Read the model definition and answer for the solid it produces. Units are mm, in the model's axes. Face numbers are marked on the shaded views. A direction names the side the tool comes from. Coordinates: 2 decimals unless noted, no trailing zeros. Loops run counter-clockwise (first coordinate to the right, second up) from the corner with the lowest first, then second, coordinate; pieces in that order, holes last.
from build123d import *

# Parameters (mm, degrees)
FILLET1_R       = 0.2
FILLET2_R       = 0.4
HEX_2_DEPTH     = 2
THDSCHPAT_COUNT = 29
THDSCHPAT_PITCH = 0.689655172


with BuildPart() as part:
    # BodySke → Base-Revolve (revolve)
    with BuildSketch(Plane.XY, mode=Mode.PRIVATE) as base_revolve_sk:
        Polygon((0, 0), (0, 3.5), (4, 3.5), (4, 2), (43.61, 2), (44, 1.61), (44, 0), align=None)
    revolve(base_revolve_sk.sketch.rotate(Axis((-31.75, 0, 0), (1, 0, 0)), 90), axis=Axis((-31.75, 0, 0), (1, 0, 0)))  # turned: the seam where the file's is

    # Fillet1
    fillet1_edges = [part.edges().sort_by_distance(p)[0] for p in [
        (4, 0, -2),
    ]]
    fillet(fillet1_edges, radius=FILLET1_R)

    # Fillet2
    fillet2_edges = [part.edges().sort_by_distance(p)[0] for p in [
        (0, 0, -3.5),
    ]]
    fillet(fillet2_edges, radius=FILLET2_R)

    # Sketch2 → Hex-PreBroach (revolve, cut)
    with BuildSketch(Plane.XY, mode=Mode.PRIVATE) as hex_prebroach_sk:
        Polygon((0, 1.51), (2, 1.51), (2.871798906, 0), (0, 0), align=None)
    revolve(hex_prebroach_sk.sketch.rotate(Axis((0, 0, 0), (1, 0, 0)), 90), axis=Axis((0, 0, 0), (1, 0, 0)), mode=Mode.SUBTRACT)  # turned: the seam where the file's is

    # Sketch3 → Hex 2 (cut)
    with BuildSketch(Plane(origin=(0, 0, 0), x_dir=(0, 0.5, 0.866025404), z_dir=(-1, 0, 0))):
        Polygon((0.871798906, 1.51), (-0.871798906, 1.51), (-1.743597813, 0), (-0.871798906, -1.51), (0.871798906, -1.51), (1.743597813, 0), align=None)
    extrude(amount=-HEX_2_DEPTH, mode=Mode.SUBTRACT)

    # ThdSchSke → ThreadSchematic (revolve, cut)
    with BuildSketch(Plane.XY, mode=Mode.PRIVATE) as threadschematic_sk:
        Polygon((24, -1.61), (23.72691906, -2), (23.72691906, -2.5), (24.27308094, -2.5), (24.27308094, -2), align=None)
    threadschematic = revolve(threadschematic_sk.sketch.rotate(Axis((-3.175, 0, 0), (1, 0, 0)), 270), axis=Axis((-3.175, 0, 0), (1, 0, 0)), mode=Mode.SUBTRACT)  # turned: the seam where the file's is

    # ThdSchPat: ThreadSchematic ×29
    with Locations(*[(i * THDSCHPAT_PITCH, 0, 0) for i in range(1, THDSCHPAT_COUNT)]):
        add(threadschematic, mode=Mode.SUBTRACT)


solid = part.part
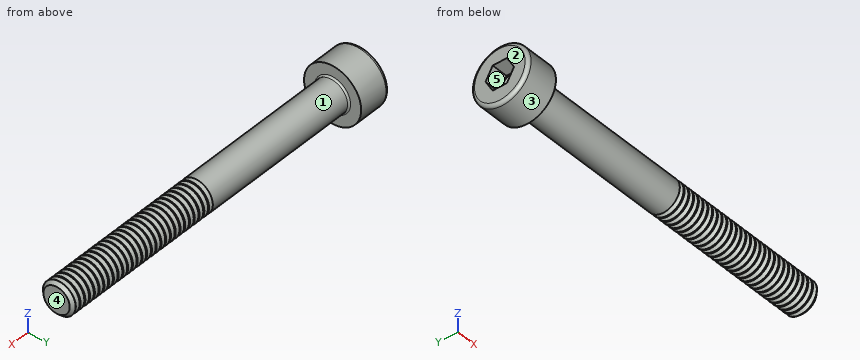
Q1. Flat-ended cylindrical pins translate along their axes: pin 1 Ø1 at (x, z) = (10, -0.5) entering from +Y; pin 2 Ø1.5 at (x, y) = (33, 1) entering from +Z; pin 3 Ø0.6 at (y, z) = (-0.5, -1) entering from -X. Find the tip coordinate at first contact, or state that the pin passes through.
Findings below:
pin 1: stops at y = 2
pin 2: stops at z = 1.98
pin 3: stops at x = 2.05
Q2. A cutting plane is placed at A-A (x = 9.5). Give the vertices of the cut face in (y, z).
Findings below:
outline: circle Ø4 at (0, 0)
Q3. Straight lines are drawn through the part: probe 1 along X at (y, z) = (-1.75, 1.25); probe 2 along Z at (x, y) = (3.5, 2.5); probe 3 along Z at (x, y) = (3, -1.25). For each, find the intervals that lie inside material, in ascending order.
Findings below:
probe 1: x = 0 to 4.01
probe 2: z = -2.45 to 2.45
probe 3: z = -3.27 to 3.27
Q4. Determine the mould class of the marked faces 3, 4 and 5 for opening direction Z: +Z half, -Z half, draft (parallel to the pull), parting line (faces both ways), or undercut.
Findings below:
face 3: parting line
face 4: draft
face 5: undercut
Q5. Which of the six approach directions +Z, -Z, +X, -X, +Y, -Y give full straight-line access (tool end or side, diameter ignored) to the marked faces 1 and 2?
Findings below:
face 1: +X
face 2: +Z, -Z, -X, +Y, -Y
